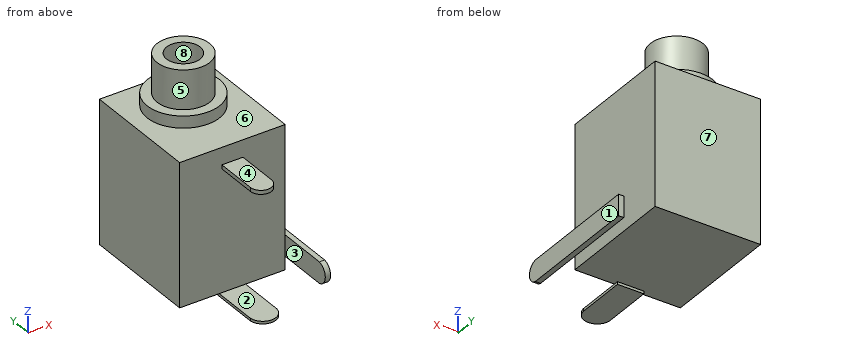
Autodesk Inventor part; units mm, degrees
ref_plane "YZ Plane" through (0, 0, 0) normal (1, 0, 0) x (0, 1, 0)
ref_plane "XZ Plane" through (0, 0, 0) normal (0, 1, 0) x (-1, 0, 0)
ref_plane "XY Plane" through (0, 0, 0) normal (0, 0, 1) x (1, 0, 0)
sketch "Эскиз1" plane through (0, 0, 0) normal (0, 1, 0) x (-1, 0, 0)
  line L0 (0, 0) -> (8, 0)
  line L1 (8, 0) -> (8, -10.8)
  line L2 (8, -10.8) -> (0, -10.8)
  line L3 (0, -10.8) -> (0, 0)
  dimension "d0" = 10.8
  dimension "d1" = 8
extrude "Выдавливание1" add sketch "Эскиз1" along normal blind 9
sketch "Эскиз2" plane through (-8, 0, 0) normal (0, 0, 1) x (1, 0, 0)
  circle A0 centre (4, 5.5) radius 2.75
  line L0 (8, 0) -> (8, 9)
  line L1 (0, 0) -> (8, 0)
  dimension "d4" = 5.5
  dimension "d5" = 4
  dimension "d6" = 5.5
extrude "Выдавливание2" add sketch "Эскиз2" along normal blind 0.9
sketch "Эскиз3" plane through (-4, 5.5, 0.9) normal (0, 0, 1) x (1, 0, 0)
  circle A0 centre (0, 0) radius 2
  point P0 (4, -5.5)
  dimension "d9" = 4
extrude "Выдавливание3" add sketch "Эскиз3" along normal blind 2.95
sketch "Эскиз4" plane through (-4, 5.5, 3.85) normal (0, 0, 1) x (1, 0, 0)
  circle A0 centre (0, 0) radius 2.75
  circle A1 centre (0, 0) radius 1.275
  point P0 (4, -5.5)
  dimension "d12" = 2.55
extrude "Выдавливание4" cut sketch "Эскиз4" against normal blind 7.9 contours A1
sketch "Эскиз5" plane through (-8, 0, 0) normal (0, 0, 1) x (1, 0, 0)
  point P0 (8, 0)
sketch "Эскиз6" plane through (0, 0, 0) normal (0, -1, 0) x (1, 0, 0)
  line L0 (-4.8, -1.3) -> (-3.2, -1.3)
  line L1 (-3.2, -1.3) -> (-3.2, -1.6)
  line L2 (-3.2, -1.6) -> (-4.8, -1.6)
  line L3 (-4.8, -1.6) -> (-4.8, -1.3)
  line L4 (0, 0) -> (0, -10.8)
  line L5 (-8, 0) -> (0, 0)
  line L6 (0, -10.8) -> (-8, -10.8)
  dimension "d15" = 1.6
  dimension "d16" = 0.3
  dimension "d17" = 3.2
  dimension "d39" = 9.2
extrude "Выдавливание5" add sketch "Эскиз6" along normal blind 4
sketch "Эскиз7" plane through (-4.8, 0, -1.3) normal (0, 0, 1) x (1, 0, 0)
  line L0 (0, 0) -> (0, -4)
  line L1 (1.6, 0) -> (1.6, -4)
  arc A0 (0, -3.2011) -> (1.6, -3.2011) centre (0.8, -3.2011) ccw
  line L2 (0, -3.2011) -> (0, -4)
  line L3 (1.6, -4) -> (0, -4)
  line L4 (1.6, -4) -> (1.6, -3.2011)
  point P0 (4.8, 0)
  point P1 (0.7588, -4)
  point P2 (0.8412, -4)
extrude "Выдавливание6" cut sketch "Эскиз7" against normal blind 4
sketch "Эскиз8" plane through (0, 0, 0) normal (1, 0, 0) x (0, 0, -1)
  line L0 (8.2, 5.5) -> (9.8, 5.5)
  line L1 (9.8, 5.5) -> (9.8, -4.5)
  line L2 (9.8, -4.5) -> (8.2, -4.5)
  line L3 (8.2, -4.5) -> (8.2, 5.5)
  line L4 (0, 9) -> (10.8, 9)
  line L5 (0, 0) -> (0, 9)
  dimension "d23" = 1.6
  dimension "d24" = 3.5
  dimension "d25" = 8.2
  dimension "d26" = 10
extrude "Выдавливание7" add sketch "Эскиз8" along normal blind 0.4
sketch "Эскиз9" plane through (0.4, 0, 0) normal (1, 0, 0) x (0, 0, -1)
  line L0 (8.2, 0) -> (8.2, -4.5)
  line L1 (9.8, -4.5) -> (9.8, 0)
  arc A0 (8.2, -3.8439) -> (9.8, -3.8337) centre (8.999, -3.6854) ccw
  line L2 (8.2, -3.8439) -> (8.2, -4.5)
  line L3 (8.2, -4.5) -> (9.8, -4.5)
  line L4 (9.8, -4.5) -> (9.8, -3.8337)
  point P0 (0, 0)
  point P1 (8.9981, -4.5)
extrude "Выдавливание8" cut sketch "Эскиз9" against normal blind 0.4
sketch "Эскиз10" plane through (0, 0, -10.8) normal (0, 0, -1) x (-1, 0, 0)
  line L0 (3, 0.35) -> (5, 0.35)
  line L1 (5, 0.35) -> (5, -4.4)
  line L2 (5, -4.4) -> (3, -4.4)
  line L3 (3, -4.4) -> (3, 0.35)
  line L4 (8, 0) -> (8, 9)
  line L5 (0, 0) -> (8, 0)
  dimension "d31" = 2
  dimension "d32" = 3
  dimension "d33" = 4.75
  dimension "d34" = 0.35
extrude "Выдавливание9" add sketch "Эскиз10" along normal blind 0.2
sketch "Эскиз11" plane through (0, 0, -11) normal (0, 0, -1) x (-1, 0, 0)
  line L0 (3, 0.35) -> (3, -4.4)
  line L1 (5, -4.4) -> (5, 0.35)
  arc A0 (3, -3.4779) -> (5, -3.4779) centre (4, -3.3967) ccw
  line L2 (3, -4.4) -> (5, -4.4)
  line L3 (3, -3.4779) -> (3, -4.4)
  line L4 (3, -4.4) -> (5, -4.4)
  line L5 (5, -4.4) -> (5, -3.4779)
  point P0 (0, 0)
  point P1 (4, -4.4)
extrude "Выдавливание10" cut sketch "Эскиз11" against normal blind 0.2
properties part number "PY-401N"
Geometry: final body of the model. Coordinates: model frame, mm. Face numbers are marked on the shaded views. A direction names the side the tool comes from. Give positions to 0.01 mm unless a question says otherwise; leave off trailing zeros. Write each loop counter-clockwise with the first axis right and the second up, starting at its lowest first coordinate (ties: lowest second). Pieces come first, ordered by that corner, then holes.
(1) Access query for the marked faces 1, 2, 3 and 4. Directions: +Z, -Z, +X, -X, +Y, -Y. A direction counts if a zero-diameter tool reaches every point of the face in a straight line with its end or side. Return the directions, or none.
(2) Mould query, pull axis Y, two halves, no side actions, for the marked faces 5, 6, 7 and 8. Classes: released by +Y, released by -Y, zero draft, split by the parting line, or undercut.
(3) Ray query, line 1 (Y direction, x = -4, z = -1.5) (3 decimals); line 2 (Y direction, x = -4, z = -0.75) (3 decimals); line 3 (Y direction, x = -5.5, z = -5.75). Return the intervals inside material, ascending.
(4) Cut plane C-C, the plane x = -4. Return loops of the section in (y, z) (3 decimals), then the cut area to 3 significant figures.
(5) Cut plane B-B, the plane y = 2.5. Return loops of the section in (x, z), then the cut area to 3 significant figures.
(6) Cut plane A-A, the plane y = -2.75. Return loops of the section in (x, z), then the cut area to 3 significant figures.
(7) Cut plane D-D, the plane z = -6. Return loops of the section in (x, y).
(8) First-contact query: P1, Ø2, axis at x = -4, y = 5.5, coming from the +Z side; P2, Ø3, axis at y = 4, z = 2, coming from the -X side; P3, Ø2, axis at x = -1, z = -3.5, coming from the -Y side. Flat tips, straight axial feed; report the tip coordinate or a pass-through.
Values follow:
1. face 1: +Z, -Z, +X, +Y, -Y
1. face 2: +X, -X, -Y
1. face 3: +Z, -Z, -X, -Y
1. face 4: +Z, +X, -X, -Y
2. face 5: split by the parting line
2. face 6: zero draft
2. face 7: released by +Y
2. face 8: undercut
3. line 1: y = -4.001 to 4.225, 6.775 to 9
3. line 2: y = 0 to 4.225, 6.775 to 9
3. line 3: y = 0 to 9
4. outline: (-4.4, -11) - (0.35, -11) - (0.35, -10.8) - (9, -10.8) - (9, 0) - (8.25, 0) - (8.25, 0.9) - (7.5, 0.9) - (7.5, 3.85) - (6.775, 3.85) - (6.775, -4.05) - (4.225, -4.05) - (4.225, 3.85) - (3.5, 3.85) - (3.5, 0.9) - (2.75, 0.9) - (2.75, 0) - (0, 0) - (0, -1.3) - (-4.001, -1.3) - (-4.001, -1.6) - (0, -1.6) - (0, -10.8) - (-4.4, -10.8) - close
4. area: 96.0 mm2
5. outline: (-8, -10.8) - (0, -10.8) - (0, -9.8) - (0.4, -9.8) - (0.4, -8.2) - (0, -8.2) - (0, 0) - (-8, 0) - close
5. area: 87.0 mm2
6. outline: (-5, -11) - (-3, -11) - (-3, -10.8) - (-5, -10.8) - close; (-4.8, -1.6) - (-3.2, -1.6) - (-3.2, -1.3) - (-4.8, -1.3) - close; (0, -9.8) - (0.4, -9.8) - (0.4, -8.2) - (0, -8.2) - close
6. area: 1.52 mm2
7. outline: (-8, 0) - (0, 0) - (0, 9) - (-8, 9) - close
8. P1: stops at z = -4.05
8. P2: stops at x = -6.71
8. P3: stops at y = 0
